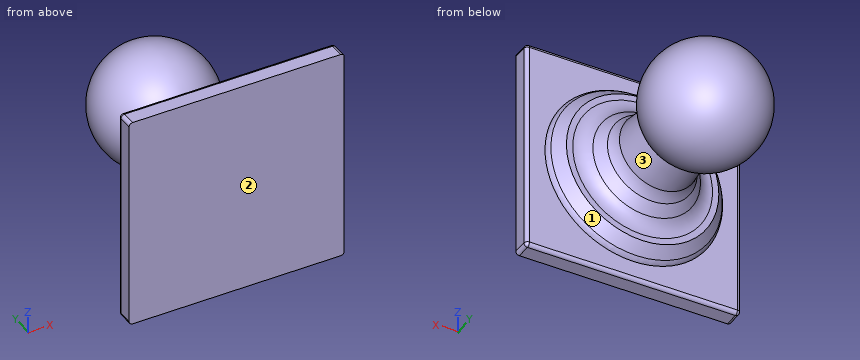
from build123d import *

# Parameters (mm, degrees)
FILLET1_R           = 1.651
FILLET2_R           = 3.048
SKETCH2_W           = 30.48
SKETCH2_H           = 30.48
BOSS_EXTRUDE1_DEPTH = 2.54
FILLET3_R           = 0.508


with BuildPart() as part:
    # Sketch1 → Revolve1 (revolve)
    with BuildSketch(Plane(origin=(0, 0, 0), x_dir=(0, 0, -1), z_dir=(1, 0, 0)), mode=Mode.PRIVATE) as revolve1_sk:
        with BuildLine():
            Line((0, 14.5542), (0, -14.5542))
            Line((0, -14.5542), (12.5603, -14.5542))
            Line((12.5603, -14.5542), (12.5603, -11.698058268))
            Line((12.5603, -11.698058268), (10.796510879, -9.7155))
            Line((10.796510879, -9.7155), (8.532673765, -9.7155))
            Line((8.532673765, -9.7155), (5.715, -6.548339963))
            Line((5.715, -6.548339963), (5.08, -0.795239963))
            ThreePointArc((5.08, -0.795239963), (8.084115709, 8.714342259), (0, 14.5542))
        make_face()
    revolve(revolve1_sk.sketch.rotate(Axis((0, 14.5542, 0), (0, -1, 0)), 180), axis=Axis((0, 14.5542, 0), (0, -1, 0)))

    # Fillet1
    fillet1_edges = [part.edges().sort_by_distance(p)[0] for p in [
        (0, -14.5542, -12.5603),
        (0, -11.698058268, -12.5603),
    ]]
    fillet(fillet1_edges, radius=FILLET1_R)

    # Fillet2
    fillet2_edges = [part.edges().sort_by_distance(p)[0] for p in [
        (0, -9.7155, -8.532673765),
        (0, -6.548339963, -5.715),
    ]]
    fillet(fillet2_edges, radius=FILLET2_R)

    # Sketch2 → Boss-Extrude1 (add)
    with BuildSketch(Plane.XZ.offset(14.5542)):
        Rectangle(SKETCH2_W, SKETCH2_H)
    extrude(amount=-BOSS_EXTRUDE1_DEPTH)

    # Fillet3
    fillet3_edges = [part.edges().sort_by_distance(p)[0] for p in [
        (-15.24, -12.0142, 0),
        (-15.24, -13.2842, -15.24),
        (0, -12.0142, 15.24),
        (-15.24, -13.2842, 15.24),
        (15.24, -12.0142, 0),
        (15.24, -13.2842, 15.24),
        (0, -12.0142, -15.24),
        (15.24, -13.2842, -15.24),
    ]]
    fillet(fillet3_edges, radius=FILLET3_R)


solid = part.part
Here's how the part is built. I have some questions about the finished solid (model axes, mm). Face numbers are marked on the shaded views. Give positions to 0.01 mm unless a question says otherwise; leave off trailing zeros. Write each loop counter-clockwise with the first axis right and the second up, starting at its lowest first coordinate (ties: lowest second). Pieces come first, ordered by that corner, then holes. Notation, with made-up numbers: (-34.75, -32.5) -> (-3.75, -32.5) arc R24 cw to (-3.75, -3.5) -> close; hole circle Ø9 at (80, 84.5). An arc over 180 degrees is marked (long way). Use one line per item in the form item = value. Start each with the question number.
1. Thinking about a two-plate mould opening in Y: for the marked faces 1, 2 and 3, which applies, +Y half, -Y half, draft (parallel to the pull), parting line (faces both ways), or undercut?
2. Will these pins go through, and if not, where does the flat tip stop? pin 1 Ø8 at (x, y) = (7.5, 1) entering from -Z; pin 2 Ø14.5 at (x, z) = (-2.5, -7) entering from +Y; pin 3 Ø5 at (x, y) = (-7.5, -7.5) entering from +Z.
3. If I drill on L1, parallel to Y at x = -2.5, z = 7; L2, parallel to Y at x = -3, z = -6; L3, parallel to Y at x = 13, z = -6, over which ranges is the centre line in solid material (lowest first)?
4. Imagine slicing it at A-A on z = -13. List the corners of the cut face in (x, y) for me, plus the area to 3 significant figures.
5. Imagine slicing it at B-B on y = 3.5. List the corners of the cut face in (x, z) for me.
Entries:
q1.face_1 = +Y half
q1.face_2 = -Y half
q1.face_3 = undercut
q2.pin_1 = -6.87
q2.pin_2 = 14.55
q2.pin_3 = 8.74
q3.L1 = -14.55 to -8.48, 1.88 to 10.19
q3.L2 = -14.55 to -7.66, 0.79 to 11.28
q3.L3 = -14.55 to -12.01
q4.outline = (-15.24, -14.55) -> (15.24, -14.55) -> (15.24, -12.52) arc R0.51 ccw to (14.73, -12.01) -> (-14.73, -12.01) arc R0.51 ccw to (-15.24, -12.52) -> close
q4.area = 77.3 mm²
q5.outline = circle Ø16.26 at (0, 0)
